from build123d import *

# Parameters (mm, degrees)
F3_R     = 2.5
F4_DEPTH = 35


with BuildPart() as f1:
    # F0 (on Top) → F1 (revolve)
    with BuildSketch(Plane.XY):
        with BuildLine():
            ThreePointArc((3, 2.75), (5.3408484106, 1.4432355034), (5.4570149341, -1.2351427503))
            Line((5.4570149341, -1.2351427503), (6.2748163897, -1.2351427503))
            ThreePointArc((6.2748163897, -1.2351427503), (6.378961338, 0.9124802881), (5.2078915499, 2.7157346895))
            ThreePointArc((5.2078915499, 2.7157346895), (4.1715222121, 3.29811093), (3, 3.5))
            Line((3, 3.5), (3, 2.75))
        make_face()
        with BuildLine():
            Line((3, 5.9120398946), (3, 3.5))
            ThreePointArc((3, 3.5), (4.1715222121, 3.29811093), (5.2078915499, 2.7157346895))
            Line((5.2078915499, 2.7157346895), (5.2078915499, 5.9120398946))
            Line((5.2078915499, 5.9120398946), (3, 5.9120398946))
        make_face()
    revolve(axis=Axis((3, -1.5105393408, 0), (0, -1, 0)))

    # F3 (on offset) → F4 (join, symmetric)
    with BuildSketch(Plane.YZ.offset(36)):
        with Locations((7.1499980986, 0)):
            Circle(F3_R)
    extrude(amount=F4_DEPTH, both=True)


with BuildPart() as f1_1:
    # F5: moved
    add(f1.part.moved(Location((0, -7.2, 0))))

    # F6 (on Front) → F7 (revolve)
    with BuildSketch(Plane.XZ):
        with BuildLine():
            ThreePointArc((68.8586309552, -2.7275545988), (71.1994793659, -4.0343190953), (71.3156458893, -6.712697349))
            Line((71.3156458893, -6.712697349), (72.133447345, -6.712697349))
            ThreePointArc((72.133447345, -6.712697349), (72.2115181091, -4.4734889968), (70.9155485965, -2.64575485))
            ThreePointArc((70.9155485965, -2.64575485), (69.9399960368, -2.148793634), (68.8586309552, -1.9775545988))
            Line((68.8586309552, -1.9775545988), (68.8586309552, -2.7275545988))
        make_face()
        with BuildLine():
            Line((68.8586309552, 0.4344852958), (68.8586309552, -1.9775545988))
            ThreePointArc((68.8586309552, -1.9775545988), (69.9399960368, -2.148793634), (70.9155485965, -2.64575485))
            Line((70.9155485965, -2.64575485), (70.9155485965, 0.4344852958))
            Line((70.9155485965, 0.4344852958), (68.8586309552, 0.4344852958))
        make_face()
    revolve(axis=Axis((68.8586309552, 0, -3.7275545988), (0, 0, 1)))


solid = f1_1.part
Source: CAD feature listing. Evaluate the final solid. Frame: model axes, mm. A direction names the side the tool comes from. Give positions to 0.01 mm unless a question says otherwise; leave off trailing zeros. Order: outer loops, then holes, each group sorted by start corner. A loop starts at its lowest first (then second) coordinate and runs counter-clockwise, first axis right, second up. Notation, with made-up numbers: (73, -0.5) -> (126, -0.5) arc R14 ccw to (126, 7.5) -> close; hole circle Ø1 at (35, 57.5). An arc over 180 degrees is marked (long way). Write item = value, one per line.
Item 1: Section query D-D (z = -4.5). Output: boundary loops of the cut face in (x, y), then the cut area to 3 significant figures.
Check result:
outline = circle Ø6.72 at (68.86, 0); hole circle Ø5.14 at (68.86, 0)
area = 14.7 mm²
Item 2: Section query C-C (x = 49.5). Output: boundary loops of the cut face in (y, z), then the cut area to 3 significant figures.
Check result:
outline = circle Ø5 at (-0.05, 0)
area = 19.6 mm²
Item 3: Contact query for flat-ended pins moving along their axis: pin 1 (1.5 mm diameter, centred on x = 7.5, z = -0.5, fed in from -Y); pin 2 (6 mm diameter, centred on x = 64, y = -6.5, fed in from +Z); pin 3 (2 mm diameter, centred on y = -5, z = 1, fed in from -X); pin 4 (4 mm diameter, centred on y = -1, z = 1, fed in from -X). Output: stop coordinate, or through.
Check result:
pin_1 = -2.55
pin_2 = through
pin_3 = -0.2
pin_4 = 0.79
Item 4: Ray query, probe 1 along Y at (x, z) = (28, 0.25); probe 2 along Z at (x, y) = (64.5, -1); probe 3 along Z at (x, y) = (13.5, 1.5). Return the intervals inside material, ascending.
Check result:
probe_1 = -2.54 to 2.44
probe_2 = -2.31 to 2.31
probe_3 = -1.96 to 1.96
Item 5: Mould query, pull axis Z, two halves, no side actions, for faces 4 (the face through (69.964, 1.734, -2.275)), 5 (the face through (1, 0, 0)), 6 (the face through (0.794, -3.219, 0.097)). Classes: +Z half, -Z half, draft (parallel to the pull), parting line (faces both ways), or undercut.
Check result:
face_4 = undercut
face_5 = draft
face_6 = parting line
Item 6: Section query B-B (z = 0). Output: boundary loops of the cut face in (x, y), then the cut area to 3 significant figures.
Check result:
outline = (-0.27, -8.44) -> (0.54, -8.44) arc R2.75 cw (long way) to (5.46, -8.44) -> (6.27, -8.44) arc R3.5 ccw to (5.21, -4.48) -> (5.21, -2.55) -> (71, -2.55) -> (71, 2.45) -> (1, 2.45) -> (1, -1.29) -> (0.79, -1.29) -> (0.79, -4.48) arc R3.5 ccw to start
area = 366 mm²
Item 7: Set-up query: faces 1 (the face through (71, 0, 0)), 2 (the face through (66, 1, -6.713)), 3 (the face through (36.49, -0.38, 2.48)). Return all of +Z, -Z, +X, -X, +Y, -Y with unobstructed straight access to the full face (end or side cutting, diameter ignored); none if empty.
Check result:
face_1 = +Z, +X, +Y, -Y
face_2 = -Z, +X, -X, +Y, -Y
face_3 = none
Item 8: Section query A-A (y = 0). Output: boundary loops of the cut face in (x, z).
Check result:
outline = (1, -2.5) -> (66.8, -2.5) -> (66.8, -2.65) arc R3.5 ccw to (65.58, -6.71) -> (66.4, -6.71) arc R2.75 cw (long way) to (71.32, -6.71) -> (72.13, -6.71) arc R3.5 ccw to (70.92, -2.65) -> (70.92, -2.5) -> (71, -2.5) -> (71, 2.5) -> (1, 2.5) -> close
